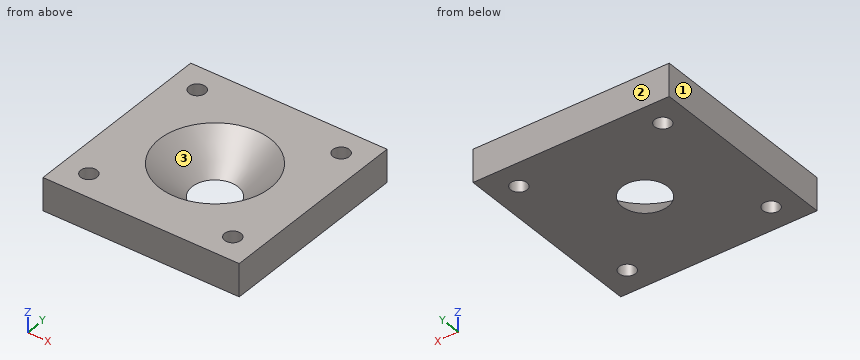
from build123d import *

# Parameters (mm, degrees)
F0_W     = 38.1
F0_H     = 38.1
F1_DEPTH = 6.35
F2_R     = 4.445
F3_DEPTH = 25.4
F4_DEPTH = 6.35
F4_TAPER = -45
F5_R     = 1.5875
F6_DEPTH = 25.4


with BuildPart() as f1:
    # F0 (on Top) → F1 (new body)
    with BuildSketch(Plane.XY):
        Rectangle(F0_W, F0_H)
    extrude(amount=F1_DEPTH)

    # F2 (on Top) → F3 (cut)
    with BuildSketch(Plane.XY):
        Circle(F2_R)
    extrude(amount=F3_DEPTH, mode=Mode.SUBTRACT)

    # F2 (on Top) → F4 (cut)
    with BuildSketch(Plane.XY):
        Circle(F2_R)
    extrude(amount=F4_DEPTH, taper=F4_TAPER, mode=Mode.SUBTRACT)

    # F5 (on Top) → F6 (cut)
    with BuildSketch(Plane.XY):
        with Locations((13.97, -13.97)):
            Circle(F5_R)
        with Locations((13.97, 13.97)):
            Circle(F5_R)
        with Locations((-13.97, -13.97)):
            Circle(F5_R)
        with Locations((-13.97, 13.97)):
            Circle(F5_R)
    extrude(amount=F6_DEPTH, mode=Mode.SUBTRACT)


solid = f1.part
Geometry check sheet. Reference: the model listing, model coordinates, mm. Face numbers are marked on the shaded views. Round coordinates to 2 decimals unless told otherwise and drop trailing zeros. Order: outer loops, then holes, each group sorted by start corner. A loop starts at its lowest first (then second) coordinate and runs counter-clockwise, first axis right, second up. Notation, with made-up numbers: M -11.75,59.25 L 36.25,59.25 A29 ccw 36.25,79.25 Z; hole C 3.5,57.5 d5. An arc over 180 degrees is marked long. Answer in a Markdown table with one row per item. Add a question column.
Item 1: Sectioned sample at D-D, the plane x = 0. Enter the section's corners in (y, z) (3 decimals).
Item 2: Sectioned sample at C-C, the plane z = 5.25. State how many separate pieces and enclosed holes the cut face has, plus the area to 3 significant figures.
Item 3: Depth check by flat-ended pin: pin 1 Ø3 at (x, y) = (-13.97, -13.97) entering from -Z. Enter the tip coordinate at first touch or a pass-through.
Item 4: Sectioned sample at A-A, the plane y = -13.97. Enter the section's corners in (x, z).
Item 5: Material ranges on L1, parallel to Y at x = 13.97, z = 5; L2, parallel to X at y = -13, z = 5.5, recorded low to high. Write a range as [from, to].
Item 6: Draft check along X on the marked faces 1, 2 and 3. Enter one of: released by +X, released by -X, zero draft, split by the parting line, or undercut.
Filled in:
| question | item | result |
|---|---|---|
| 1 | outline | M -19.05,0 L -4.445,0 L -10.795,6.35 L -19.05,6.35 Z; M 4.445,0 L 19.05,0 L 19.05,6.35 L 10.795,6.35 Z |
| 2 | separate pieces | 1 |
| 2 | enclosed holes | 5 |
| 2 | area | 1,120 mm² |
| 3 | pin 1 | passes through |
| 4 | outline | M -19.05,0 L -15.56,0 L -15.56,6.35 L -19.05,6.35 Z; M -12.38,0 L 12.38,0 L 12.38,6.35 L -12.38,6.35 Z; M 15.56,0 L 19.05,0 L 19.05,6.35 L 15.56,6.35 Z |
| 5 | L1 | y = [-19.05, -15.56], [-12.38, 12.38], [15.56, 19.05] |
| 5 | L2 | x = [-19.05, -15.23], [-12.71, 12.71], [15.23, 19.05] |
| 6 | face 1 | released by -X |
| 6 | face 2 | zero draft |
| 6 | face 3 | undercut |
